```python
from build123d import *

# Parameters (mm, degrees)
F0_W     = 914.4
F0_H     = 609.6
F1_DEPTH = 914.4
F2_T     = -25.4
F3_W     = 609.6
F3_H     = 25.4
F4_DEPTH = 863.6


with BuildPart() as f1:
    # F0 (on Top) → F1 (new body)
    with BuildSketch(Plane.XY):
        with Locations((-1.154758, 4.566898)):
            Rectangle(F0_W, F0_H)
    extrude(amount=F1_DEPTH)

    # F2
    f2_openings = [f1.faces().sort_by_distance(p)[0] for p in [
        (-1.154758, 4.566898, 0),
        (-1.154758, -300.233102, 457.2),
        (-1.154758, 309.366898, 457.2),
    ]]
    offset(amount=F2_T, openings=f2_openings)

    # F3 (on face) → F4 (join, through all)
    with BuildSketch(Plane.YZ.offset(-432.954758)):
        with Locations((4.566898, 181.854316)):
            Rectangle(F3_W, F3_H)
    extrude(amount=F4_DEPTH)


solid = f1.part
```
Part model, mm, in its own coordinate system. A direction names the side the tool comes from. Coordinates: 2 decimals unless noted, no trailing zeros. Order: outer loops, then holes, each group sorted by start corner. A loop starts at its lowest first (then second) coordinate and runs counter-clockwise, first axis right, second up. Notation, with made-up numbers: (-35, 6) -> (-26, 6) arc R36 cw to (-26, 42) -> close; hole circle Ø3 at (-11, -39.5). An arc over 180 degrees is marked (long way). Put each result on its own line as item: value. Start each with the question number.
(1) Band-saw the part on B-B (x = 303.5). Give the cut face in (y, z).
(2) Which spindle directions (+Z, -Z, +X, -X, +Y, -Y) get a long thin tool onto all of the face, cutting with end or side? Do faces 5 (the face through (-432.955, 0, 83)), 6 (the face through (-7, 9, 889)), 7 (the face through (456.045, 0, 451)). Say none if no direction does.
(3) Band-saw the part on C-C (y = -151). Give the cut face in (x, z), then the cut area to 3 significant figures.
(4) Mould opens along Z. For faces 1 (the face through (-7, 0, 194.554)), 2 (the face through (-7, 0, 169.154)), 3 (the face through (430.645, 0, 83)), 4 (the face through (-432.955, 0, 537)) say: pulls with the +Z half, pulls with the -Z half, needs draft (parallel to the pull), parting line crosses it, or undercut.
(5) Probe line 1 along Z through (x, y) = (291, 245.5); line 2 along X through (y, z) = (97, 115.5). List the from-to ranges inside material, lowest first. Write a range as [from, to].
(6) Pin check, flat tip, straight feed: pin 1 Ø10 at (x, y) = (170.5, -100.5) entering from -Z. Stop position of the tip, or through.
(7) Band-saw the part on A-A (z = 425.5). Give the cut face in (x, y).
Determined:
1. outline: (-300.23, 169.15) -> (309.37, 169.15) -> (309.37, 194.55) -> (-300.23, 194.55) -> close; (-300.23, 889) -> (309.37, 889) -> (309.37, 914.4) -> (-300.23, 914.4) -> close
2. face 5: -Z, +Y, -Y
2. face 6: +Y, -Y
2. face 7: +Z, -Z, +X, +Y, -Y
3. outline: (-458.35, 0) -> (-432.95, 0) -> (-432.95, 169.15) -> (430.65, 169.15) -> (430.65, 0) -> (456.05, 0) -> (456.05, 914.4) -> (-458.35, 914.4) -> close; hole (-432.95, 194.55) -> (430.65, 194.55) -> (430.65, 889) -> (-432.95, 889) -> close
3. area: 90,300 mm²
4. face 1: undercut
4. face 2: pulls with the -Z half
4. face 3: needs draft
4. face 4: undercut
5. line 1: z = [169.15, 194.55], [889, 914.4]
5. line 2: x = [-458.35, -432.95], [430.65, 456.05]
6. pin 1: stops at z = 169.15
7. outline: (-458.35, -300.23) -> (-432.95, -300.23) -> (-432.95, 309.37) -> (-458.35, 309.37) -> close; (430.65, -300.23) -> (456.05, -300.23) -> (456.05, 309.37) -> (430.65, 309.37) -> close
